The drawing under review shows one solid part. Ordinate dimensions are in mm from its lowest x, y, z. A direction names the side the tool comes from. Coordinates: 2 decimals unless noted, no trailing zeros. Order: outer loops, then holes, each group sorted by start corner. A loop starts at its lowest first (then second) coordinate and runs counter-clockwise, first axis right, second up. Notation, with made-up numbers: (86, -1.75) -> (96, -1.75) arc R19 ccw to (96, 22.25) -> close; hole circle Ø3 at (80, -34.75). An arc over 180 degrees is marked (long way). Write item = value, one per line.
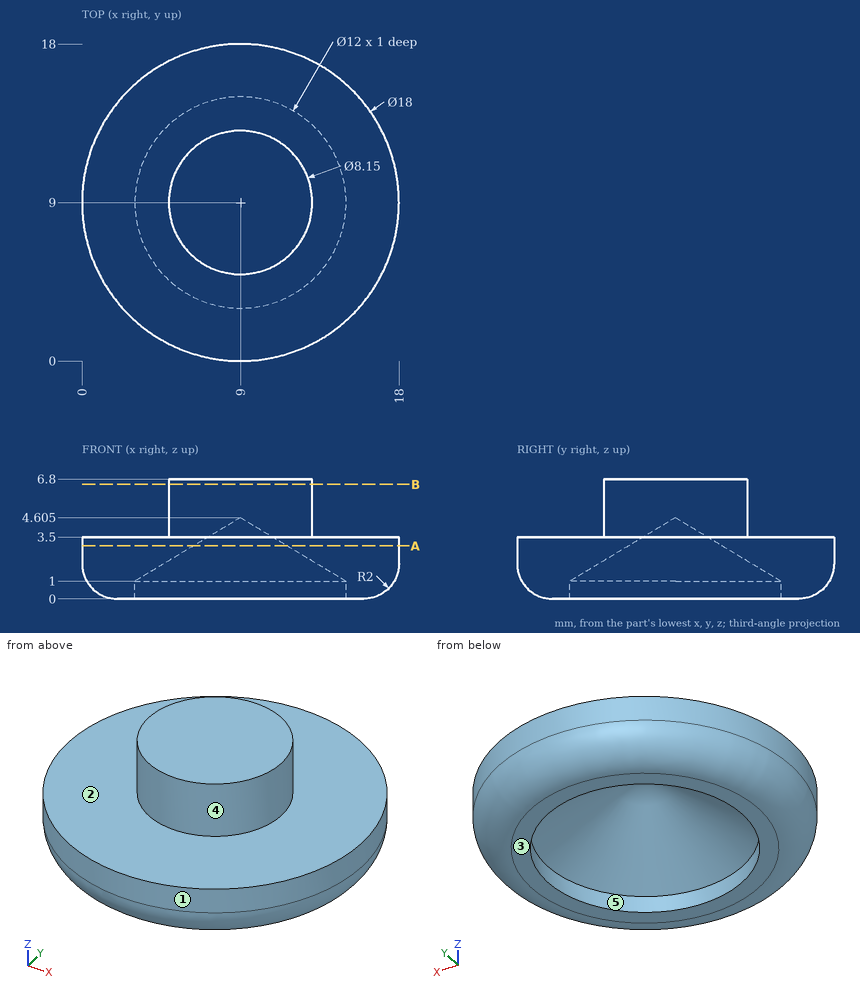
(1) We need section B-B (z = 6.5). Write out the cut boundary in (x, y) (3 decimals), and give its area (3 significant figures).
Report:
outline = circle Ø8.15 at (9, 9)
area = 52.2 mm²
(2) For the marked faces 1 and 2, list the 3-axis set-ups (+Z, -Z, +X, -X, +Y, -Y) from which the entire face can be reached by the end or side of a thin tool; tool diameter is ignored.
Report:
face_1 = +Z, -Z
face_2 = +Z
(3) We need section A-A (z = 3). Write out the cut boundary in (x, y).
Report:
outline = circle Ø18 at (9, 9); hole circle Ø5.34 at (9, 9)
(4) For L1, parallel to Y at x = 8.25, z = 1.5 (1 decimal); L2, parallel to Y at x = 9, z = 0.3; L3, parallel to Z at x = 7.25, y = 2.5, list the stretches that pass through material, from the lowest coordinate up.
Report:
L1 = 0.1 to 3.9, 14.1 to 17.9
L2 = 0.95 to 3, 15 to 17.05
L3 = 0 to 3.5
(5) The part is to be moulded in two halves that separate along X. For the marked faces 3, 4 and 5, say which applies: released by +X, released by -X, zero draft, split by the parting line, or undercut.
Report:
face_3 = zero draft
face_4 = split by the parting line
face_5 = undercut
(6) Insertion check: pin 1 (1 mm diameter, centred on x = 15.5, z = 1.5, fed in from -Y); pin 2 (4 mm diameter, centred on y = 15, z = 2, fed in from +X); pin 3 (1 mm diameter, centred on x = 9.5, y = 2.5, fed in from +Z). Each pin has a flat end and moves straight along its axis. Give the tip position at first contact, or say it passes through.
Report:
pin_1 = 2.35
pin_2 = 17.06
pin_3 = 3.5
